For this review, take the finished solid that the model builds, in its own axes (mm). Round coordinates to 2 decimals unless told otherwise and drop trailing zeros. Write each loop counter-clockwise with the first axis right and the second up, starting at its lowest first coordinate (ties: lowest second). Pieces come first, ordered by that corner, then holes. Notation, with made-up numbers: M 81.25,56.25 L 126.25,56.25 A19 cw 126.25,90.25 Z; hole C -35.5,-20 d7. An arc over 180 degrees is marked long. Use one line per item in the form item = value. Start each with the question number.
Item 1: For line 1 (Z direction, x = -89.5, y = -2.5); line 2 (X direction, y = -11, z = -16.5); line 3 (Z direction, x = -120, y = -3.5), list the stretches that pass through material, from the lowest coordinate up. Write a range as [from, to].
Item 2: Add section B-B (z = 30). State the section outline as (x, y) points, and give its area (3 significant figures).
Item 3: Add section A-A (y = -5.75). State the section outline as (x, z) points (1 decimal).
from build123d import *

# Parameters (mm, degrees)
F0_W     = 101.6
F0_H     = 215.9
F0_R     = 1.5875
F1_DEPTH = 12.7
F2_R     = 25.4
F3_R     = 25.4
F4_R     = 25.4
F5_R     = 25.4


with BuildPart() as f1:
    # F0 (on Front) → F1 (new body)
    with BuildSketch(Plane.XZ):
        with Locations((-90.611439, -64.121174)):
            Rectangle(F0_W, F0_H)
        with Locations((-90.611439, -111.363955)):
            Circle(F0_R, mode=Mode.SUBTRACT)
        with Locations((-90.611439, -151.368955)):
            Circle(F0_R, mode=Mode.SUBTRACT)
        with Locations((-90.611439, -16.748955)):
            Circle(F0_R, mode=Mode.SUBTRACT)
    extrude(amount=F1_DEPTH)

    # F2
    f2_edges = [f1.edges().sort_by_distance(p)[0] for p in [
        (-141.411439, -6.35, 43.828826),
    ]]
    fillet(f2_edges, radius=F2_R)

    # F3
    f3_edges = [f1.edges().sort_by_distance(p)[0] for p in [
        (-39.811439, -6.35, 43.828826),
    ]]
    fillet(f3_edges, radius=F3_R)

    # F4
    f4_edges = [f1.edges().sort_by_distance(p)[0] for p in [
        (-141.411439, -6.35, -172.071174),
    ]]
    fillet(f4_edges, radius=F4_R)

    # F5
    f5_edges = [f1.edges().sort_by_distance(p)[0] for p in [
        (-39.811439, -6.35, -172.071174),
    ]]
    fillet(f5_edges, radius=F5_R)


solid = f1.part
Calculated:
q1.line_1 = [-172.07, -152.5], [-150.24, -112.5], [-110.23, -17.88], [-15.62, 43.83]
q1.line_2 = [-141.41, -92.18], [-89.04, -39.81]
q1.line_3 = [-171.76, 43.51]
q2.outline = M -138.62,-12.7 L -42.6,-12.7 L -42.6,0 L -138.62,0 Z
q2.area = 1,220 mm^2
q3.outline = M -141.4,-146.7 A25.4 ccw -116,-172.1 L -65.2,-172.1 A25.4 ccw -39.8,-146.7 L -39.8,18.4 A25.4 ccw -65.2,43.8 L -116,43.8 A25.4 ccw -141.4,18.4 Z; hole C -90.6,-151.4 d3.2; hole C -90.6,-111.4 d3.2; hole C -90.6,-16.7 d3.2
